Design review of the part built by this model. Coordinates are the model's own, in mm. Face numbers are marked on the shaded views. A direction names the side the tool comes from. Round coordinates to 2 decimals unless told otherwise and drop trailing zeros. Loops run counter-clockwise (first coordinate to the right, second up) from the corner with the lowest first, then second, coordinate; pieces in that order, holes last. Notation, with made-up numbers: (59, 50) -> (104, 50) arc R16 cw to (104, 68) -> close; hole circle Ø4 at (-4, 34.5). An arc over 180 degrees is marked (long way). Answer as CSV lines item,"result". Start each with the question number.
(1) To check wall thickness, follow line 1 (Y direction, x = 52, z = 2.35); line 2 (Y direction, x = 52.75, z = 1.7); line 3 (X direction, y = 30, z = 2.1). State the ranges of each line that lie inside material, in increasing order. Write a range as from..to.
(2) Take a section at A-A, the plane y = 30. Write out the cut boundary in (x, z).
(3) Take a section at B-B, the plane x = 52. Write out the cut boundary in (y, z).
(4) Take a section at D-D, the plane x = 45.5. Write out the cut boundary in (y, z).
(5) Draft analysis for pull direction Y (two halves, no side actions). For the marked faces 1, 2 and 3, state which applies: +Y half, -Y half, draft (parallel to the pull), parting line (faces both ways), or undercut.
(6) Take a section at C-C, the plane z = 2.45. Write out the cut boundary in (x, y).
(7) Machinability: for the marked faces 4, 5 and 6, which of the approach directions +Z, -Z, +X, -X, +Y, -Y give a long, thin tool a straight path to every point of the face, cutting with its end or side? Answer none if there is none.
(8) For P1, Ø0.9, axis at y = 12, z = 1, coming from the -X side; P2, Ø1.5, axis at y = 12, z = 1, coming from the +X side; P3, Ø1.5, axis at x = 57, z = 1.5, coming from the +Y side, all flat-tipped, find the tip position at first contact; note any pin that passes through.
from build123d import *

# Parameters (mm, degrees)
CORTE_EXTERIOR_R        = 1.05
CORTE_EXTERIOR_R_2      = 3.5
SALIENTE_EXTRUIR1_DEPTH = 3
CORTAR_EXTRUIR1_DEPTH   = 1


with BuildPart() as part:
    # Corte exterior → Saliente-Extruir1 (new body)
    with BuildSketch(Plane.XY):
        Polygon((49.5, 10.5), (54.5, 10.5), (54.5, 13.5), (59.5, 13.5), (59.5, 29.5), (59.5, 46.5), (54.5, 46.5), (54.5, 49.5), (49.5, 49.5), (49.5, 46.5), (44.5, 46.5), (44.5, 23.5), (44.5, 13.5), (49.5, 13.5), align=None)
        with Locations((52, 40.672229454)):
            Circle(CORTE_EXTERIOR_R, mode=Mode.SUBTRACT)
        with Locations((52, 19.327770547)):
            Circle(CORTE_EXTERIOR_R, mode=Mode.SUBTRACT)
        with Locations((52, 30)):
            Circle(CORTE_EXTERIOR_R_2, mode=Mode.SUBTRACT)
    extrude(amount=SALIENTE_EXTRUIR1_DEPTH)

    # Grabado Superficie → Cortar-Extruir1 (cut)
    with BuildSketch(Plane.XY):
        with BuildLine():
            Line((48.730825792, 28.75), (50, 15.7))
            ThreePointArc((50, 15.7), (52, 13.7), (54, 15.7))
            Line((54, 15.7), (55.269174208, 28.75))
            ThreePointArc((55.269174208, 28.75), (52, 26.5), (48.730825792, 28.75))
        make_face()
        with BuildLine():
            Line((55.269174208, 31.25), (53.990313411, 44.196602453))
            ThreePointArc((53.990313411, 44.196602453), (51.901579532, 45.997576885), (50, 44))
            Line((50, 44), (48.730825792, 31.25))
            ThreePointArc((48.730825792, 31.25), (52, 33.5), (55.269174208, 31.25))
        make_face()
    extrude(amount=CORTAR_EXTRUIR1_DEPTH, mode=Mode.SUBTRACT)


solid = part.part
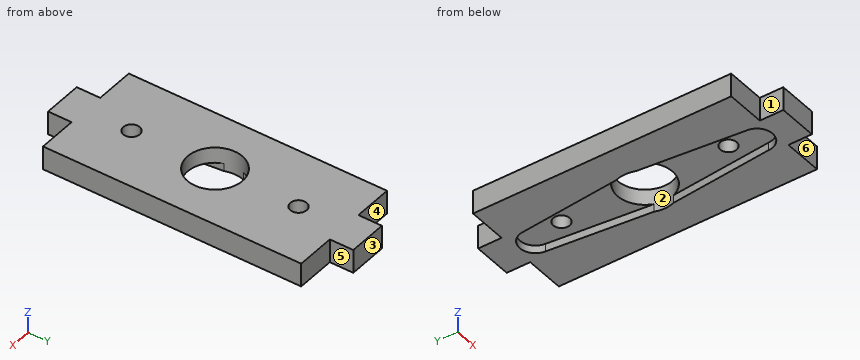
The answers:
1,line 1,"10.5..18.28, 20.38..26.5, 33.5..39.62, 41.72..49.5"
1,line 2,"10.5..18.59, 20.06..26.58, 33.42..39.94, 41.41..49.5"
1,line 3,"44.5..48.5, 55.5..59.5"
2,outline,"(44.5, 0) -> (48.5, 0) -> (48.5, 3) -> (44.5, 3) -> close; (55.5, 0) -> (59.5, 0) -> (59.5, 3) -> (55.5, 3) -> close"
3,outline,"(10.5, 0) -> (13.7, 0) -> (13.7, 1) -> (18.28, 1) -> (18.28, 3) -> (10.5, 3) -> close; (20.38, 1) -> (26.5, 1) -> (26.5, 3) -> (20.38, 3) -> close; (33.5, 1) -> (39.62, 1) -> (39.62, 3) -> (33.5, 3) -> close; (41.72, 1) -> (46, 1) -> (46, 0) -> (49.5, 0) -> (49.5, 3) -> (41.72, 3) -> close"
4,outline,"(13.5, 0) -> (46.5, 0) -> (46.5, 3) -> (13.5, 3) -> close"
5,face 1,"draft"
5,face 2,"undercut"
5,face 3,"+Y half"
6,outline,"(44.5, 13.5) -> (49.5, 13.5) -> (49.5, 10.5) -> (54.5, 10.5) -> (54.5, 13.5) -> (59.5, 13.5) -> (59.5, 46.5) -> (54.5, 46.5) -> (54.5, 49.5) -> (49.5, 49.5) -> (49.5, 46.5) -> (44.5, 46.5) -> close; hole circle Ø7 at (52, 30); hole circle Ø2.1 at (52, 19.33); hole circle Ø2.1 at (52, 40.67)"
7,face 4,"+Z, -Z, -X, +Y"
7,face 5,"+Z, -Z, +X, +Y"
7,face 6,"+Z, -Z, +X, -Y"
8,P1,"x = 49.5"
8,P2,"x = 54.5"
8,P3,"y = 46.5"
